Autodesk Inventor part; units mm, degrees
ref_plane "YZ Plane" through (0, 0, 0) normal (1, 0, 0) x (0, 1, 0)
ref_plane "XZ Plane" through (0, 0, 0) normal (0, 1, 0) x (-1, 0, 0)
ref_plane "XY Plane" through (0, 0, 0) normal (0, 0, 1) x (1, 0, 0)
sketch "Sketch1" plane through (0, 0, 0) normal (0, 1, 0) x (-1, 0, 0)
  line L0 (0, 0) -> (-101.6, 0)
  line L1 (-101.6, 0) -> (-101.6, 38.1)
  line L2 (-101.6, 38.1) -> (0, 38.1)
  line L3 (0, 38.1) -> (0, 0)
  line L4 (0, 19.05) -> (-101.6, 19.05) construction
  line L5 (0, 9.2781) -> (-25.4, 9.2781) construction
  line L6 (-25.4, 9.2781) -> (-50.8, 9.2781) construction
  line L7 (-50.8, 9.2781) -> (-76.2, 9.2781) construction
  line L8 (-76.2, 9.2781) -> (-101.6, 9.2781) construction
  line L9 (-101.6, 9.2781) -> (-101.6, 9.2781) construction
  circle A0 centre (-25.4, 19.05) radius 2.5797
  circle A1 centre (-50.8, 19.05) radius 2.5797
  circle A2 centre (-76.2, 19.05) radius 2.5797
  dimension "d0" = 101.6
  dimension "d1" = 38.1
  dimension "d2" = 25.4
  dimension "d3" = 25.4
  dimension "d4" = 25.4
  dimension "d5" = 25.4
  dimension "d6" = 5.1594
  dimension "d7" = 5.1594
  dimension "d8" = 5.1594
extrude "Extrusion1" add sketch "Sketch1" along normal blind 5.08
sketch "Sketch2" plane through (101.6, 0, 0) normal (0, 0, -1) x (-1, 0, 0)
  line L0 (0, 5.08) -> (101.6, 5.08)
  line L1 (101.6, 5.08) -> (0, 5.08)
  line L2 (0, 5.08) -> (0, -38.1)
  line L3 (0, -38.1) -> (101.6, -38.1)
  line L4 (101.6, -38.1) -> (101.6, 5.08)
  point P0 (101.6, 0)
  dimension "d11" = 43.18
extrude "Extrusion2" add sketch "Sketch2" along normal blind 5.08
properties part number "jig proto1"
Geometry: final body of the model. Coordinates: model frame, mm. A direction names the side the tool comes from. Round coordinates to 2 decimals unless told otherwise and drop trailing zeros. Order: outer loops, then holes, each group sorted by start corner. A loop starts at its lowest first (then second) coordinate and runs counter-clockwise, first axis right, second up. Notation, with made-up numbers: (-2, 48) - (26, 48) arc R19 cw to (26, 52) - close; hole circle Ø6 at (-13.5, 13). An arc over 180 degrees is marked (long way). Write item = value, one per line. Start each with the question number.
Q1. Access query for faces 1 (the flat face through (52, -38.1, -3)), 2 (the flat face through (52, -19, 0)). Directions: +Z, -Z, +X, -X, +Y, -Y. A direction counts if a zero-diameter tool reaches every point of the face in a straight line with its end or side. Return the directions, or none.
Q2. Pin query (flat end, axial travel): pin 1 (6 mm diameter, centred on x = 50.8, z = 19.05, fed in from +Y); pin 2 (19 mm diameter, centred on x = 69, z = 23.5, fed in from -Y); pin 3 (8 mm diameter, centred on x = 56.5, y = -22, fed in from +Z). Return the tip coordinate at first contact, or that it passes through.
Q3. Cut plane A-A on z = 19.05. Return the cut outline in (x, y), and give its area (4 significant figures).
Q4. Ray query, line 1 (X direction, y = 1, z = 19); line 2 (Z direction, x = 50.8, y = 3.9); line 3 (Y direction, x = 82, z = 36.5). Return the intervals inside material, ascending. Write a range as from..to.
Q5. Pull-direction query (Z, two-part tool) for faces 3 (the flat face through (101.6, 1, 7)), 4 (the cylindrical face through (27.447, 2.504, 20.62)), 5 (the flat face through (52, -16, -5.08)), 6 (the cylindrical face through (75.01, 2.5, 21.34)); classes: +Z half, -Z half, draft (parallel to the pull), parting line (faces both ways), or undercut.
Q6. Cut plane C-C on x = 56.5. Return the cut outline in (y, z), and give its area (3 significant figures).
Q7. Cut plane D-D on z = 25.5. Return the cut outline in (x, y), and give its area (3 significant figures).
Q8. Cut plane B-B on x = 25.4. Return the cut outline in (y, z), and give its area (3 significant figures).
Outcome:
q1.face_1 = +Z, -Z, +X, -X, -Y
q1.face_2 = +Z, +X, -X, -Y
q2.pin_1 = 5.08
q2.pin_2 = 0
q2.pin_3 = 0
q3.outline = (0, 0) - (22.82, 0) - (22.82, 5.08) - (0, 5.08) - close; (27.98, 0) - (48.22, 0) - (48.22, 5.08) - (27.98, 5.08) - close; (53.38, 0) - (73.62, 0) - (73.62, 5.08) - (53.38, 5.08) - close; (78.78, 0) - (101.6, 0) - (101.6, 5.08) - (78.78, 5.08) - close
q3.area = 437.5 mm^2
q4.line_1 = 0..22.82, 27.98..48.22, 53.38..73.62, 78.78..101.6
q4.line_2 = -5.08..16.47, 21.63..38.1
q4.line_3 = 0..5.08
q5.face_3 = draft
q5.face_4 = undercut
q5.face_5 = -Z half
q5.face_6 = undercut
q6.outline = (-38.1, -5.08) - (5.08, -5.08) - (5.08, 38.1) - (0, 38.1) - (0, 0) - (-38.1, 0) - close
q6.area = 413 mm^2
q7.outline = (0, 0) - (101.6, 0) - (101.6, 5.08) - (0, 5.08) - close
q7.area = 516 mm^2
q8.outline = (-38.1, -5.08) - (5.08, -5.08) - (5.08, 16.47) - (0, 16.47) - (0, 0) - (-38.1, 0) - close; (0, 21.63) - (5.08, 21.63) - (5.08, 38.1) - (0, 38.1) - close
q8.area = 387 mm^2
